```python
from build123d import *

# Parameters (mm, degrees)
F0_R     = 2.6
F1_DEPTH = 12
F3_W     = 20.1
F3_H     = 8
F4_DEPTH = 30.001
F2_W     = 10.05
F2_H     = 8
F5_DEPTH = 46.001
F7_DEPTH = 5


# Not quite as in the source:
# - a fillet or chamfer that OpenCascade refuses, or shapes differently, is made with other operations: its cross-section is extruded or revolved along the edge and cut away or added


with BuildPart() as f1:
    # F0 (on Top) → F1 (new body)
    with BuildSketch(Plane.XY):
        Polygon((0, -46), (0, 14), (-30, 14), (-30, -14), (-14, -46), align=None)
        with Locations((-20.5, -20.5)):
            Circle(F0_R, mode=Mode.SUBTRACT)
    extrude(amount=F1_DEPTH)

    # F3 (on face) → F4 (cut, through all)
    with BuildSketch(Plane(origin=(-30, 0, 0), x_dir=(0, -1, 0), z_dir=(-1, 0, 0))):
        with Locations((0, 8)):
            Rectangle(F3_W, F3_H)
        Polygon((0, 0.8), (-0.8, 0), (0.8, 0), align=None)
    extrude(amount=-F4_DEPTH, mode=Mode.SUBTRACT)

    # F2 (on face) → F5 (cut, through all)
    with BuildSketch(Plane.XZ.offset(46)):
        with Locations((-5.025, 8)):
            Rectangle(F2_W, F2_H)
        Polygon((-0.8, 0), (0, 0), (0, 0.8), align=None)
    extrude(amount=-F5_DEPTH, mode=Mode.SUBTRACT)

    # F6 (on face) → F7 (cut)
    with BuildSketch(Plane.XY):
        Polygon((-15.9270442062, -21.725319812), (-17.1523640182, -17.1523640182), (-21.725319812, -15.9270442062), (-25.0729557938, -19.274680188), (-23.8476359818, -23.8476359818), (-19.274680188, -25.0729557938), align=None)
    extrude(amount=F7_DEPTH, mode=Mode.SUBTRACT)

    # F8: F1 across plane


with BuildPart() as f1_1:
    add(f1.part)
    add(f1.part.mirror(Plane.YZ))

    # F9: chamfer of 2 on 2 edges, made by hand


with BuildPart() as f9_tool2:
    # F9_s3 → F9_t4 (revolve)
    with BuildSketch(Plane.XZ.offset(20.5)):
        Polygon((17.9, 7), (15.9, 5), (17.9, 5), align=None)
    revolve(axis=Axis((20.5, -20.5, 5), (0, 0, 1)))

    split(bisect_by=Plane(origin=(20.291464501, -5.4370815263, 0), x_dir=(0, 0, 1), z_dir=(0.9659258263, -0.2588190451, 0)), keep=Keep.TOP)

    split(bisect_by=Plane(origin=(-2.8991378029, -2.8991378029, 0), x_dir=(0, 0, 1), z_dir=(0.7071067812, 0.7071067812, 0)), keep=Keep.TOP)

    split(bisect_by=Plane(origin=(5.4370815263, -20.291464501, 0), x_dir=(0, 0, 1), z_dir=(0.2588190451, -0.9659258263, 0)), keep=Keep.TOP)

    split(bisect_by=Plane(origin=(7.5593976961, -28.2120562766, 0), x_dir=(0, 0, 1), z_dir=(-0.2588190451, 0.9659258263, 0)), keep=Keep.TOP)

    split(bisect_by=Plane(origin=(2.8991378029, 2.8991378029, 0), x_dir=(0, 0, 1), z_dir=(-0.7071067812, -0.7071067812, 0)), keep=Keep.TOP)

    split(bisect_by=Plane(origin=(28.2120562766, -7.5593976961, 0), x_dir=(0, 0, 1), z_dir=(-0.9659258263, 0.2588190451, 0)), keep=Keep.TOP)


with BuildPart() as f1_2:
    add(f1_1.part)

    # F9_t1: cut F9_tool2
    add(f9_tool2.part, mode=Mode.SUBTRACT)


with BuildPart() as f9_tool12:
    # F9_s13 → F9_t14 (revolve)
    with BuildSketch(Plane.XZ.offset(20.5)):
        Polygon((-17.9, 7), (-15.9, 5), (-17.9, 5), align=None)
    revolve(axis=Axis((-20.5, -20.5, 5), (0, 0, -1)))

    split(bisect_by=Plane(origin=(-20.291464501, -5.4370815263, 0), x_dir=(0, 0, 1), z_dir=(-0.9659258263, -0.2588190451, 0)), keep=Keep.TOP)

    split(bisect_by=Plane(origin=(2.8991378029, -2.8991378029, 0), x_dir=(0, 0, 1), z_dir=(-0.7071067812, 0.7071067812, 0)), keep=Keep.TOP)

    split(bisect_by=Plane(origin=(-5.4370815263, -20.291464501, 0), x_dir=(0, 0, 1), z_dir=(-0.2588190451, -0.9659258263, 0)), keep=Keep.TOP)

    split(bisect_by=Plane(origin=(-7.5593976961, -28.2120562766, 0), x_dir=(0, 0, 1), z_dir=(0.2588190451, 0.9659258263, 0)), keep=Keep.TOP)

    split(bisect_by=Plane(origin=(-2.8991378029, 2.8991378029, 0), x_dir=(0, 0, 1), z_dir=(0.7071067812, -0.7071067812, 0)), keep=Keep.TOP)

    split(bisect_by=Plane(origin=(-28.2120562766, -7.5593976961, 0), x_dir=(0, 0, 1), z_dir=(0.9659258263, 0.2588190451, 0)), keep=Keep.TOP)


with BuildPart() as f1_3:
    add(f1_2.part)

    # F9_t11: cut F9_tool12
    add(f9_tool12.part, mode=Mode.SUBTRACT)


solid = f1_3.part
```
Work out the finished part from the listing and answer in its coordinate system (mm). A direction names the side the tool comes from. Give positions to 0.01 mm unless a question says otherwise; leave off trailing zeros. Loops run counter-clockwise (first coordinate to the right, second up) from the corner with the lowest first, then second, coordinate; pieces in that order, holes last. Notation, with made-up numbers: (67, -22.75) -> (89, -22.75) arc R8 ccw to (89, -11.75) -> close; hole circle Ø3 at (38.25, 30.25). An arc over 180 degrees is marked (long way). Write item = value, one per line. Start each with the question number.
(1) Which of the six approach directions +Z, -Z, +X, -X, +Y, -Y give full straight-line access (tool end or side, diameter ignored) to faces 1 (the flat face through (0, 12, 12)), 2 (the flat face through (-17.6, -23.4, 2.7)), 3 (the flat face through (-10.05, -28, 8))?
(2) Given pin 1 Ø3 at (y, z) = (0, 6.5) entering from +X; pin 2 Ø4 at (y, z) = (-36.5, 5.5) entering from +X, each flat-ended and moving along its own axis, determine where each tip first touches the part or whether it passes through.
(3) Find section C-C on y = -37.5. Give the vertices of the cut face in (x, z).
(4) Find section B-B on z = 2.75. Give the vertices of the cut face in (x, y), and give its area (3 significant figures).
(5) The mould has two halves that part along Y. Classify faces 4 (the flat face through (0, 7, 0)), 5 (the flat face through (0, -11, 4)), 6 (the flat face through (0, 14, 6)): +Y half, -Y half, draft (parallel to the pull), parting line (faces both ways), or undercut.
(6) Find the intervals of material crossed by probe 1 along X at (y, z) = (-12.5, 6); probe 2 along X at (y, z) = (-20.5, 10.7); probe 3 along Y at (x, z) = (-21, 8.5), in increasing order. Write a range as from..to.
(7) Find section A-A on z = 8.5. Give the vertices of the cut face in (x, y).
(8) Find section D-D on x = -20.5. Give the vertices of the cut face in (y, z), and give its area (3 significant figures).
From the geometry:
q1.face_1 = +Z, +X, -X, +Y, -Y
q1.face_2 = -Z
q1.face_3 = +Z, -Y
q2.pin_1 = through
q2.pin_2 = 19.75
q3.outline = (-18.25, 0) -> (-0.8, 0) -> (0, 0.8) -> (0.8, 0) -> (18.25, 0) -> (18.25, 12) -> (10.05, 12) -> (10.05, 4) -> (-10.05, 4) -> (-10.05, 12) -> (-18.25, 12) -> close
q4.outline = (-30, -14) -> (-14, -46) -> (14, -46) -> (30, -14) -> (30, 14) -> (-30, 14) -> close; hole (-25.07, -19.27) -> (-23.85, -23.85) -> (-19.27, -25.07) -> (-15.93, -21.73) -> (-17.15, -17.15) -> (-21.73, -15.93) -> close; hole (15.93, -21.73) -> (19.27, -25.07) -> (23.85, -23.85) -> (25.07, -19.27) -> (21.73, -15.93) -> (17.15, -17.15) -> close
q4.area = 2,970 mm^2
q5.face_4 = draft
q5.face_5 = undercut
q5.face_6 = +Y half
q6.probe_1 = -30..-10.05, 10.05..30
q6.probe_2 = -26.75..-23.1, -17.9..-10.05, 10.05..17.9, 23.1..26.75
q6.probe_3 = -32..-23.05, -17.95..-10.05, 10.05..14
q7.outline = (-30, -14) -> (-14, -46) -> (-10.05, -46) -> (-10.05, -10.05) -> (-30, -10.05) -> close; (-30, 10.05) -> (30, 10.05) -> (30, 14) -> (-30, 14) -> close; (10.05, -46) -> (14, -46) -> (30, -14) -> (30, -10.05) -> (10.05, -10.05) -> close; hole circle Ø5.2 at (-20.5, -20.5); hole circle Ø5.2 at (20.5, -20.5)
q8.outline = (-33, 0) -> (-24.74, 0) -> (-24.74, 5.36) -> (-23.1, 7) -> (-23.1, 12) -> (-33, 12) -> close; (-17.9, 7) -> (-16.26, 5.36) -> (-16.26, 0) -> (-0.8, 0) -> (0, 0.8) -> (0.8, 0) -> (14, 0) -> (14, 12) -> (10.05, 12) -> (10.05, 4) -> (-10.05, 4) -> (-10.05, 12) -> (-17.9, 12) -> close
q8.area = 320 mm^2
